For this review, take the finished solid that the model builds, in its own axes (mm). Face numbers are marked on the shaded views. Round coordinates to 2 decimals unless told otherwise and drop trailing zeros. Loops run counter-clockwise (first coordinate to the right, second up) from the corner with the lowest first, then second, coordinate; pieces in that order, holes last.
1. Consider section B-B on y = 37.5. State the section outline as (x, z) points.
2. Clearance check with flat-ended pins moving along their axes: pin 1 Ø4 at (x, z) = (0, 0) entering from +Y; pin 2 Ø4 at (x, y) = (1, 47) entering from +Z; pin 3 Ø1 at (y, z) = (71.5, -2) entering from -X; pin 4 Ø1.5 at (y, z) = (58.5, -1.5) entering from -X. State where each tip first meets the part, or that it passes through.
3. Draft analysis for pull direction X (two halves, no side actions). For the marked faces 1 and 2, state which applies: released by +X, released by -X, zero draft, split by the parting line, or undercut.
4. Consider section C-C on z = -3. State the section outline as (x, y) points, then the cut area to 3 significant figures.
5. Consider section A-A on y = 68. State the section outline as (x, z) points, then the cut area to 3 significant figures.
6. To check wall thickness, follow line 1 along Z through (x, y) = (-1.25, 5); line 2 along Z through (x, y) = (0.25, 21.5); line 3 along X through (y, z) = (15, 3.25). State the ranges of each line that lie inside material, in increasing order.
from build123d import *

# Parameters (mm, degrees)
BOSS_EXTRUDE1_DEPTH       = 80
BOSS_EXTRUDE1_DEPTH_BACK  = 0.0001
SKETCH1_R                 = 4
M5X0_8_TAPPED_HOLE1_D     = 4.2
M5X0_8_TAPPED_HOLE1_DEPTH = 14
M5X0_8_TAPPED_HOLE1_TIP   = 1.2618073
M5X0_8_TAPPED_HOLE2_D     = 4.2
M5X0_8_TAPPED_HOLE2_DEPTH = 14
M5X0_8_TAPPED_HOLE2_TIP   = 1.2618073


with BuildPart() as part:
    # Sketch1 → Boss-Extrude1 (new, two sides: drawn at the far end of the back side and taken through both)
    with BuildSketch(Plane(origin=(0, 0, 0), x_dir=(1, 0, 0), z_dir=(0, 1, 0)).offset(-BOSS_EXTRUDE1_DEPTH_BACK)):
        with Locations(Location((0, 0, 0), (0, 0, 270))):
            Circle(SKETCH1_R)
    extrude(amount=BOSS_EXTRUDE1_DEPTH + BOSS_EXTRUDE1_DEPTH_BACK)

    # M5x0.8 Tapped Hole1
    with Locations(Plane(origin=(0, 80, 0), x_dir=(1, 0, 0), z_dir=(0, 1, 0))):
        with Locations((0, 0)):
            Hole(M5X0_8_TAPPED_HOLE1_D / 2, depth=M5X0_8_TAPPED_HOLE1_DEPTH)
            with Locations((0, 0, -(M5X0_8_TAPPED_HOLE1_DEPTH + M5X0_8_TAPPED_HOLE1_TIP / 2))):  # 118° drill point
                Cone(0, M5X0_8_TAPPED_HOLE1_D / 2, M5X0_8_TAPPED_HOLE1_TIP, mode=Mode.SUBTRACT)

    # M5x0.8 Tapped Hole2
    with Locations(Plane(origin=(0, -0.0001, 0), x_dir=(-1, 0, 0), z_dir=(0, -1, 0))):
        with Locations((0, 0)):
            Hole(M5X0_8_TAPPED_HOLE2_D / 2, depth=M5X0_8_TAPPED_HOLE2_DEPTH)
            with Locations((0, 0, -(M5X0_8_TAPPED_HOLE2_DEPTH + M5X0_8_TAPPED_HOLE2_TIP / 2))):  # 118° drill point
                Cone(0, M5X0_8_TAPPED_HOLE2_D / 2, M5X0_8_TAPPED_HOLE2_TIP, mode=Mode.SUBTRACT)


solid = part.part
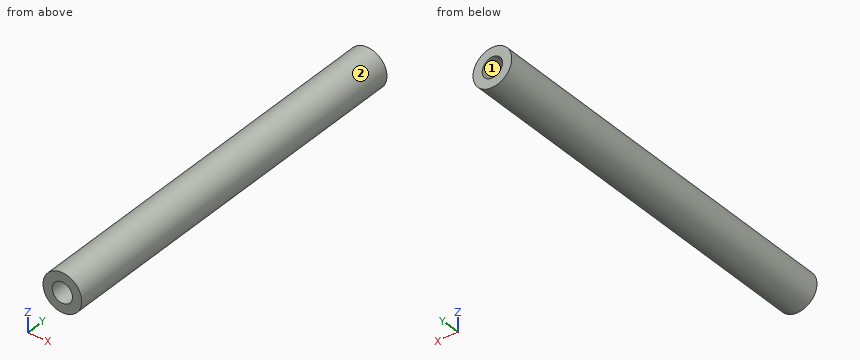
Resolved:
1. outline: circle Ø8 at (0, 0)
2. pin 1: stops at y = 65.94
2. pin 2: stops at z = 4
2. pin 3: stops at x = -3.71
2. pin 4: stops at x = -3.93
3. face 1: undercut
3. face 2: split by the parting line
4. outline: (-2.65, 0) - (2.65, 0) - (2.65, 80) - (-2.65, 80) - close
4. area: 423 mm2
5. outline: circle Ø8 at (0, 0); hole circle Ø4.2 at (0, 0)
5. area: 36.4 mm2
6. line 1: z = -3.8 to -1.69, 1.69 to 3.8
6. line 2: z = -3.99 to 3.99
6. line 3: x = -2.33 to 2.33
